```python
from build123d import *

# Parameters (mm, degrees)
CROQUIS1_R              = 30
CROQUIS1_R_2            = 19
SALIENTE_EXTRUIR1_DEPTH = 30
CROQUIS2_W              = 80
CROQUIS2_H              = 80
SALIENTE_EXTRUIR2_DEPTH = 80
CROQUIS4_R              = 30
CROQUIS4_R_2            = 19
SALIENTE_EXTRUIR4_DEPTH = 30
SALIENTE_EXTRUIR6_START = -30
CROQUIS6_R              = 30
CROQUIS6_R_2            = 19
SALIENTE_EXTRUIR6_DEPTH = 30


with BuildPart() as part:
    # Croquis1 → Saliente-Extruir1 (new body)
    with BuildSketch(Plane.XY):
        Circle(CROQUIS1_R)
        Circle(CROQUIS1_R_2, mode=Mode.SUBTRACT)
    extrude(amount=SALIENTE_EXTRUIR1_DEPTH)

    # Croquis2 → Saliente-Extruir2 (add)
    with BuildSketch(Plane.XY):
        Rectangle(CROQUIS2_W, CROQUIS2_H)
    extrude(amount=-SALIENTE_EXTRUIR2_DEPTH)

    # Croquis4 → Saliente-Extruir4 (add)
    with BuildSketch(Plane(origin=(0, 40, 0), x_dir=(1, 0, 0), z_dir=(0, 1, 0))):
        with Locations(Location((0, 40, 0), (0, 0, 270))):
            Circle(CROQUIS4_R)
        with Locations(Location((0, 40, 0), (0, 0, 270))):
            Circle(CROQUIS4_R_2, mode=Mode.SUBTRACT)
    extrude(amount=SALIENTE_EXTRUIR4_DEPTH)

    # Croquis6 → Saliente-Extruir6 (add)
    with BuildSketch(Plane.XY.offset(-80).offset(SALIENTE_EXTRUIR6_START)):
        with Locations(Location((0, 0, 0), (0, 0, 180))):
            Circle(CROQUIS6_R)
        Circle(CROQUIS6_R_2, mode=Mode.SUBTRACT)
    extrude(amount=SALIENTE_EXTRUIR6_DEPTH)


solid = part.part
```
Input: part model. Units: mm. Frame: model coordinates. A direction names the side the tool comes from. Give positions to 0.01 mm unless a question says otherwise; leave off trailing zeros. Write each loop counter-clockwise with the first axis right and the second up, starting at its lowest first coordinate (ties: lowest second). Pieces come first, ordered by that corner, then holes. Notation, with made-up numbers: (13.5, -12) - (63.5, -12) arc R18 cw to (63.5, -2) - close; hole circle Ø2 at (-14.5, -38). An arc over 180 degrees is marked (long way). Write item = value, one per line. Start each with the question number.
1. First-contact query: pin 1 Ø23 at (x, y) = (0, 0) entering from -Z; pin 2 Ø2 at (x, y) = (7.5, -3) entering from +Z; pin 3 Ø6 at (x, z) = (-11.5, 14) entering from -Y. Flat tips, straight axial feed; report the tip coordinate or a pass-through.
2. Section query C-C, the plane z = -40. Output: boundary loops of the cut face in (x, y), then the cut area to 3 significant figures.
3. Access query for faces 1 (the cylindrical face through (-18.548, 54.79, -44.119)), 2 (the cylindrical face through (8.767, -16.856, 14.79)), 3 (the cylindrical face through (-16.128, -25.296, -95.21)). Directions: +Z, -Z, +X, -X, +Y, -Y. A direction counts if a zero-diameter tool reaches every point of the face in a straight line with its end or side. Return the directions, or none.
4. Ray query, L1, parallel to Z at x = -0.5, y = 50.5; L2, parallel to X at y = 63, z = -40. Return the intervals inside material, ascending.
5. Mould query, pull axis Y, two halves, no side actions, for faces 4 (the flat face through (0, 0, 0)), 5 (the flat face through (0, 40, -40)), 6 (the flat face through (0, 20, -110)), 7 (the cylindrical face through (-29.97, 1.32, 14.79)). Classes: released by +Y, released by -Y, zero draft, split by the parting line, or undercut.
6. Section query D-D, the plane y = 58.5. Output: boundary loops of the cut face in (x, z), then the cut area to 3 significant figures.
7. Section query A-A, the plane x = 0. Output: boundary loops of the cut face in (y, z).
8. Section query B-B, the plane y = 0. Output: boundary loops of the cut face in (x, z), then the cut area to 3 significant figures.
Check sheet entries:
q1.pin_1 = -80
q1.pin_2 = 0
q1.pin_3 = -28.77
q2.outline = (-40, -40) - (40, -40) - (40, 40) - (30, 40) - (30, 70) - (19, 70) - (19, 40) - (-19, 40) - (-19, 70) - (-30, 70) - (-30, 40) - (-40, 40) - close
q2.area = 7,060 mm2
q3.face_1 = +Y
q3.face_2 = +Z
q3.face_3 = -Z
q4.L1 = -70 to -58.99, -21.01 to -10
q4.L2 = -30 to -19, 19 to 30
q5.face_4 = undercut
q5.face_5 = released by +Y
q5.face_6 = zero draft
q5.face_7 = split by the parting line
q6.outline = circle Ø60 at (0, -40); hole circle Ø38 at (0, -40)
q6.area = 1,690 mm2
q7.outline = (-40, -80) - (-30, -80) - (-30, -110) - (-19, -110) - (-19, -80) - (19, -80) - (19, -110) - (30, -110) - (30, -80) - (40, -80) - (40, -70) - (70, -70) - (70, -59) - (40, -59) - (40, -21) - (70, -21) - (70, -10) - (40, -10) - (40, 0) - (30, 0) - (30, 30) - (19, 30) - (19, 0) - (-19, 0) - (-19, 30) - (-30, 30) - (-30, 0) - (-40, 0) - close
q8.outline = (-40, -80) - (-30, -80) - (-30, -110) - (-19, -110) - (-19, -80) - (19, -80) - (19, -110) - (30, -110) - (30, -80) - (40, -80) - (40, 0) - (30, 0) - (30, 30) - (19, 30) - (19, 0) - (-19, 0) - (-19, 30) - (-30, 30) - (-30, 0) - (-40, 0) - close
q8.area = 7,720 mm2
